Verification items for the finished model (mm, model axes). A direction names the side the tool comes from. Coordinates: 2 decimals unless noted, no trailing zeros. Write each loop counter-clockwise with the first axis right and the second up, starting at its lowest first coordinate (ties: lowest second). Pieces come first, ordered by that corner, then holes. Notation, with made-up numbers: (6, 10) -> (41, 10) arc R20 ccw to (41, 34) -> close; hole circle Ø2 at (7.25, -12.5). An arc over 180 degrees is marked (long way). Answer in a Markdown table with one row per item.
```python
from build123d import *

# Parameters (mm, degrees)
SKETCH1_R           = 1
BOSS_EXTRUDE1_DEPTH = 1
SKETCH2_R           = 1.5
SKETCH2_R_2         = 1
BOSS_EXTRUDE2_DEPTH = 5


with BuildPart() as part:
    # Sketch1 → Boss-Extrude1 (new body)
    with BuildSketch(Plane.XY):
        with BuildLine():
            ThreePointArc((-6, 2.828427125), (-10, 0), (-6, -2.828427125))
            ThreePointArc((-6, -2.828427125), (0, -1.798989873), (6, -2.828427125))
            ThreePointArc((6, -2.828427125), (10, 0), (6, 2.828427125))
            ThreePointArc((6, 2.828427125), (0, 1.798989873), (-6, 2.828427125))
        make_face()
        with Locations((-7, 0)):
            Circle(SKETCH1_R, mode=Mode.SUBTRACT)
        with Locations((7, 0)):
            Circle(SKETCH1_R, mode=Mode.SUBTRACT)
    boss_extrude1 = extrude(amount=BOSS_EXTRUDE1_DEPTH)

    # Sketch2 → Boss-Extrude2 (add)
    with BuildSketch(Plane.XY.offset(1)):
        with Locations((-7, 0)):
            Circle(SKETCH2_R)
        with Locations((-7, 0)):
            Circle(SKETCH2_R_2, mode=Mode.SUBTRACT)
        with Locations((7, 0)):
            Circle(SKETCH2_R)
        with Locations((7, 0)):
            Circle(SKETCH2_R_2, mode=Mode.SUBTRACT)
    extrude(amount=BOSS_EXTRUDE2_DEPTH)

    # Mirror1: Boss-Extrude1 across plane
    add(boss_extrude1.mirror(Plane.XY.offset(3)))


solid = part.part
```
1. Go/stop test with flat-tipped pins: pin 1 (2 mm diameter, centred on x = 5, z = 4.5, fed in from +Y); pin 2 (1.6 mm diameter, centred on x = -7, y = 0, fed in from -Z). Record where each tip stops, or that it passes through.
Findings below:
| item | result |
|---|---|
| pin 1 | stops at y = 2.78 |
| pin 2 | passes through |
2. Release check for a two-part mould opening along Y. For faces 1 (the face through (10, -0.1, 5.5)), 2 (the face through (0, 0, 0)), 3 (the face through (-7.8, -0.6, 3)) record: released by +Y, released by -Y, zero draft, split by the parting line, or undercut.
Findings below:
| item | result |
|---|---|
| face 1 | split by the parting line |
| face 2 | zero draft |
| face 3 | undercut |
3. Sectioned sample at B-B, the plane x = 7. Record the cut outline in (y, z), and give its area (3 significant figures).
Findings below:
| item | result |
|---|---|
| outline | (-3, 0) -> (-1, 0) -> (-1, 6) -> (-3, 6) -> (-3, 5) -> (-1.5, 5) -> (-1.5, 1) -> (-3, 1) -> close; (1, 0) -> (3, 0) -> (3, 1) -> (1.5, 1) -> (1.5, 5) -> (3, 5) -> (3, 6) -> (1, 6) -> close |
| area | 12.0 mm² |
4. Access from +Z, -Z, +X, -X, +Y, -Y to the whole of each face (thin tool, end or side, straight path). Record for faces 4 (the face through (6.2, -0.6, 3)), 5 (the face through (-8.5, 0.07, 2.97)).
Findings below:
| item | result |
|---|---|
| face 4 | +Z, -Z |
| face 5 | none |
5. Sectioned sample at D-D, the plane y = -1.25. Record the cut outline in (x, z).
Findings below:
| item | result |
|---|---|
| outline | (-9.73, 0) -> (9.73, 0) -> (9.73, 1) -> (7.83, 1) -> (7.83, 5) -> (9.73, 5) -> (9.73, 6) -> (-9.73, 6) -> (-9.73, 5) -> (-7.83, 5) -> (-7.83, 1) -> (-9.73, 1) -> close; hole (-6.17, 1) -> (6.17, 1) -> (6.17, 5) -> (-6.17, 5) -> close |
6. Sectioned sample at A-A, the plane y = 0. Record the cut outline in (x, z).
Findings below:
| item | result |
|---|---|
| outline | (-10, 0) -> (-8, 0) -> (-8, 6) -> (-10, 6) -> (-10, 5) -> (-8.5, 5) -> (-8.5, 1) -> (-10, 1) -> close; (-6, 0) -> (6, 0) -> (6, 6) -> (-6, 6) -> close; (8, 0) -> (10, 0) -> (10, 1) -> (8.5, 1) -> (8.5, 5) -> (10, 5) -> (10, 6) -> (8, 6) -> close; hole (-5.5, 1) -> (5.5, 1) -> (5.5, 5) -> (-5.5, 5) -> close |
7. Material ranges on probe 1 along Z at (x, y) = (-2.25, -0.75); probe 2 along Y at (x, z) = (-7, 3.9); probe 3 along Y at (x, z) = (7, 0.75), recorded low to high. Write a range as from..to.
Findings below:
| item | result |
|---|---|
| probe 1 | z = 0..1, 5..6 |
| probe 2 | y = -1.5..-1, 1..1.5 |
| probe 3 | y = -3..-1, 1..3 |
8. Sectioned sample at C-C, the plane z = 0.75. Record the cut outline in (x, y).
Findings below:
| item | result |
|---|---|
| outline | (-6, -2.83) arc R18 cw to (6, -2.83) arc R3 ccw (long way) to (6, 2.83) arc R18 cw to (-6, 2.83) arc R3 ccw (long way) to start; hole circle Ø2 at (-7, 0); hole circle Ø2 at (7, 0) |
